```python
from build123d import *

# Parameters (mm, degrees)
SKETCH_1_R      = 1.45
SKETCH_1_R_2    = 1.95
EXTRUDE_1_DEPTH = 3
FILLET_2_R      = 3


with BuildPart() as part:
    # 草图1 → 凸台-拉伸1 (new body)
    with BuildSketch(Plane(origin=(0, 0, 0), x_dir=(1, 0, 0), z_dir=(0, 1, 0))):
        Polygon((-17.5, -7.5), (-17.5, 7.5), (17.5, 7.5), (17.5, -7.5), (7.5, -7.5), (7.5, -28.5), (-7.5, -28.5), (-7.5, -7.5), align=None)
        with Locations(Location((0, -14.5, 0), (0, 0, 270))):
            Circle(SKETCH_1_R, mode=Mode.SUBTRACT)
        with Locations(Location((0, -21.5, 0), (0, 0, 270))):
            Circle(SKETCH_1_R, mode=Mode.SUBTRACT)
        with Locations(Location((-7.5, 0, 0), (0, 0, 270))):
            Circle(SKETCH_1_R_2, mode=Mode.SUBTRACT)
        with Locations(Location((7.5, 0, 0), (0, 0, 90))):
            Circle(SKETCH_1_R_2, mode=Mode.SUBTRACT)
    extrude(amount=EXTRUDE_1_DEPTH)

    # 圆角2
    fillet_2_edges = [part.edges().sort_by_distance(p)[0] for p in [
        (17.5, 1.5, 7.5),
        (7.5, 1.5, 7.5),
        (7.5, 1.5, 28.5),
        (-7.5, 1.5, 28.5),
        (-7.5, 1.5, 7.5),
        (-17.5, 1.5, 7.5),
        (-17.5, 1.5, -7.5),
        (17.5, 1.5, -7.5),
    ]]
    fillet(fillet_2_edges, radius=FILLET_2_R)


solid = part.part
```
Check sheet for the modelled part. Datum: model origin and axes. Units: mm. A direction names the side the tool comes from. Coordinates: 2 decimals unless noted, no trailing zeros. Loops run counter-clockwise (first coordinate to the right, second up) from the corner with the lowest first, then second, coordinate; pieces in that order, holes last.
1) Access from +Z, -Z, +X, -X, +Y, -Y to the whole of each face (thin tool, end or side, straight path). Record for faces 4 (the face through (-7.5, 1, 18)), 5 (the face through (-5.567, 1.479, -0.254)), 6 (the face through (13, 1, 7.5)).
2) Sectioned sample at C-C (y = 0.5). Record the boundary of the cut face in (x, z).
3) Material ranges on probe 1 along X at (y, z) = (0.7, 0); probe 2 along X at (y, z) = (0.65, 1); probe 3 along X at (y, z) = (1.7, 13), recorded low to high.
4) Gauge pin test, flat ends, axial feed: pin 1 (1.5 mm diameter, centred on x = -7.5, z = -2.5, fed in from -Y); pin 2 (0.9 mm diameter, centred on y = 1, z = 18.5, fed in from +X); pin 3 (1.5 mm diameter, centred on x = 12.5, y = 2, fed in from +Z); pin 4 (1.5 mm diameter, centred on x = 10, y = 1.5, fed in from +Z). Record the tip position at first contact, or that the pin passes through.
5) Release check for a two-part mould opening along Z. For faces 1 (the face through (0.44, 1.48, 22.88)), 2 (the face through (0, 0, 6)), 3 (the face through (-8.4, 1.52, 8.36)) record: released by +Z, released by -Z, zero draft, split by the parting line, or undercut.
6) Sectioned sample at A-A (z = 0). Record the boundary of the cut face in (x, y), and give its area (3 significant figures).
7) Sectioned sample at B-B (x = 0). Record the boundary of the cut face in (y, z), and give its area (3 significant figures).
8) Sectioned sample at D-D (z = 14.5). Record the boundary of the cut face in (x, y), and give its area (3 significant figures).
Check sheet entries:
1. face 4: +Z, -X, +Y, -Y
1. face 5: +Y, -Y
1. face 6: +Z, +X, +Y, -Y
2. outline: (-17.5, -4.5) arc R3 ccw to (-14.5, -7.5) - (14.5, -7.5) arc R3 ccw to (17.5, -4.5) - (17.5, 4.5) arc R3 ccw to (14.5, 7.5) - (10.5, 7.5) arc R3 cw to (7.5, 10.5) - (7.5, 25.5) arc R3 ccw to (4.5, 28.5) - (-4.5, 28.5) arc R3 ccw to (-7.5, 25.5) - (-7.5, 10.5) arc R3 cw to (-10.5, 7.5) - (-14.5, 7.5) arc R3 ccw to (-17.5, 4.5) - close; hole circle Ø3.9 at (-7.5, 0); hole circle Ø2.9 at (0, 14.5); hole circle Ø2.9 at (0, 21.5); hole circle Ø3.9 at (7.5, 0)
3. probe 1: x = -17.5 to -9.45, -5.55 to 5.55, 9.45 to 17.5
3. probe 2: x = -17.5 to -9.17, -5.83 to 5.83, 9.17 to 17.5
3. probe 3: x = -7.5 to 7.5
4. pin 1: stops at y = 0
4. pin 2: stops at x = 7.5
4. pin 3: stops at z = 7.5
4. pin 4: stops at z = 7.77
5. face 1: undercut
5. face 2: zero draft
5. face 3: released by +Z
6. outline: (-17.5, 0) - (-9.45, 0) - (-9.45, 3) - (-17.5, 3) - close; (-5.55, 0) - (5.55, 0) - (5.55, 3) - (-5.55, 3) - close; (9.45, 0) - (17.5, 0) - (17.5, 3) - (9.45, 3) - close
6. area: 81.6 mm2
7. outline: (0, -7.5) - (3, -7.5) - (3, 13.05) - (0, 13.05) - close; (0, 15.95) - (3, 15.95) - (3, 20.05) - (0, 20.05) - close; (0, 22.95) - (3, 22.95) - (3, 28.5) - (0, 28.5) - close
7. area: 90.6 mm2
8. outline: (-7.5, 0) - (-1.45, 0) - (-1.45, 3) - (-7.5, 3) - close; (1.45, 0) - (7.5, 0) - (7.5, 3) - (1.45, 3) - close
8. area: 36.3 mm2
